Work out the finished part from the listing and answer in its coordinate system (mm). Face numbers are marked on the shaded views. A direction names the side the tool comes from. Coordinates: 2 decimals unless noted, no trailing zeros. Loops run counter-clockwise (first coordinate to the right, second up) from the corner with the lowest first, then second, coordinate; pieces in that order, holes last. Notation, with made-up numbers: (59.5, 2.25) -> (74.5, 2.25) arc R10 cw to (74.5, 9.25) -> close; hole circle Ø9 at (40, 72.25). An arc over 180 degrees is marked (long way). Use a Markdown table: item, result. Add a question column.
```python
from build123d import *

# Parameters (mm, degrees)
PAD_DEPTH = 30


with BuildPart() as part:
    # Sketch → Pad (new body)
    with BuildSketch(Plane.YZ):
        Polygon((0, 0), (60, 0), (60, 11), (54, 11), (55, 3), (43, 3), (43, 11), (0, 11), align=None)
    extrude(amount=PAD_DEPTH)


solid = part.part
```
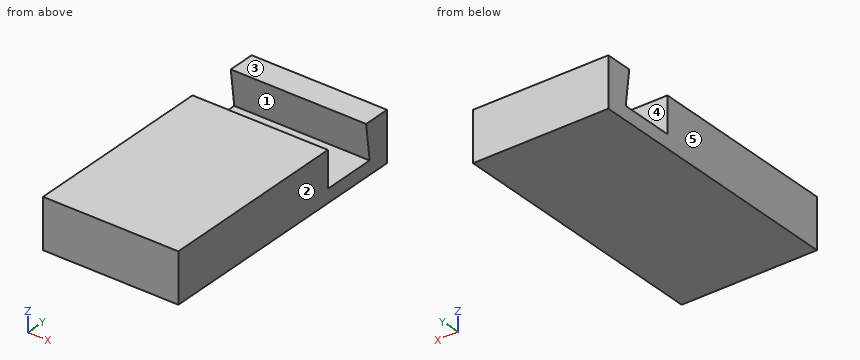
Item 1: For the marked faces 4 and 5, determine the directions among +Z, -Z, +X, -X, +Y, -Y from which every point of the face is accessible in a straight line to the end or side of a thin tool.
Item 2: Section A-A (z = 9) is taken. Determine the outline of the cut face in (x, y), then the cut area to 3 significant figures.
Item 3: Section C-C (y = 49.5) is taken. Determine the outline of the cut face in (x, z), then the cut area to 3 significant figures.
Item 4: Section B-B (x = 16.25) is taken. Determine the outline of the cut face in (y, z), then the cut area to 3 significant figures.
Item 5: For a pull along Z with two mould halves and no side action, classify the marked faces 1, 2 and 3 as +Z half, -Z half, draft (parallel to the pull), parting line (faces both ways), or undercut.
Item 6: Find the intervals of material crossed by probe 1 along Z at (x, y) = (25, 45.5); probe 2 along Y at (x, z) = (23.5, 4.75); probe 3 along Y at (x, z) = (21.5, 7.5), in increasing order.
Item 7: Section D-D (z = 5.25) is taken. Determine the outline of the cut face in (x, y), then the cut area to 3 significant figures.
Item 8: Given pin 1 (6 mm diameter, centred on x = 16, y = 48, fed in from +Z); pin 2 (10 mm diameter, centred on x = 24.5, y = 45, fed in from +Z), each flat-ended and moving along its own axis, determine where each tip first touches the part or whether it passes through.
Output:
| question | item | result |
|---|---|---|
| 1 | face 4 | +Z, +X, -X |
| 1 | face 5 | +Z, -Z, -X, +Y, -Y |
| 2 | outline | (0, 0) -> (30, 0) -> (30, 43) -> (0, 43) -> close; (0, 54.25) -> (30, 54.25) -> (30, 60) -> (0, 60) -> close |
| 2 | area | 1,460 mm2 |
| 3 | outline | (0, 0) -> (30, 0) -> (30, 3) -> (0, 3) -> close |
| 3 | area | 90.0 mm2 |
| 4 | outline | (0, 0) -> (60, 0) -> (60, 11) -> (54, 11) -> (55, 3) -> (43, 3) -> (43, 11) -> (0, 11) -> close |
| 4 | area | 568 mm2 |
| 5 | face 1 | undercut |
| 5 | face 2 | draft |
| 5 | face 3 | +Z half |
| 6 | probe 1 | z = 0 to 3 |
| 6 | probe 2 | y = 0 to 43, 54.78 to 60 |
| 6 | probe 3 | y = 0 to 43, 54.44 to 60 |
| 7 | outline | (0, 0) -> (30, 0) -> (30, 43) -> (0, 43) -> close; (0, 54.72) -> (30, 54.72) -> (30, 60) -> (0, 60) -> close |
| 7 | area | 1,450 mm2 |
| 8 | pin 1 | stops at z = 3 |
| 8 | pin 2 | stops at z = 11 |
